Could you check a few things on this model? Use its own coordinates, in mm. A direction names the side the tool comes from. Round coordinates to 2 decimals unless told otherwise and drop trailing zeros. Loops run counter-clockwise (first coordinate to the right, second up) from the corner with the lowest first, then second, coordinate; pieces in that order, holes last. Notation, with made-up numbers: M 31.25,75.5 L 74.25,75.5 A21 cw 74.25,86.5 Z; hole C 35.25,55 d8. An arc over 180 degrees is marked long. One line per item, written item: value. Start each with the question number.
Q1. Imagine slicing it at A-A (z = -1.5). Please give me the cut outline in (x, y), then the cut area to 3 significant figures.
Q2. Imagine slicing it at C-C (z = 6.5). Please give me the cut outline in (x, y), then the cut area to 3 significant figures.
Q3. Which directions (+Z, -Z, +X, -X, +Y, -Y) give clear straight access to the entire face, cutting with the end or side of a thin tool? Please do faces 5 (the face through (-5.3, -0.1, 4.2)), 6 (the face through (-2, 3, -6)), 7 (the face through (15.25, 1, 0)), 8 (the face through (-12, 4, 7)), 9 (the face through (-0.52, 0.73, 0.03)).
Q4. Thinking about a two-plate mould opening in Z: for faces 1 (the face through (-5.62, -0.22, 6)), 2 (the face through (-5.3, -0.45, 7.01)), 3 (the face through (6, 5, 4)), 4 (the face through (0, 1, -8)), which applies, released by +Z, released by -Z, zero draft, split by the parting line, or undercut?
Q5. Please list where these lines run through material, in increasing order: line 1 along X through (y, z) = (2.5, -3.25); line 2 along Z through (x, y) = (-0.5, 1.5); line 3 along X through (y, z) = (5.5, 1.5).
Q6. I'm going to push flat-ended pins straight in: pin 1 Ø1.8 at (y, z) = (6.5, -1.5) entering from -X; pin 2 Ø1.2 at (x, z) = (14.5, 4) entering from +Y; pin 3 Ø2.5 at (x, y) = (-4, 0) entering from +Z; pin 4 Ø1.5 at (x, z) = (4.5, 0.5) entering from +Y. Where does each tip first touch, or does it pass through?
Q7. Imagine slicing it at B-B (x = -5.25). Please give me the cut outline in (y, z), then the cut area to 3 significant figures.
Q8. Imagine slicing it at D-D (x = 8). Please give me the cut outline in (y, z).
from build123d import *

# Parameters (mm, degrees)
BOSS_EXTRUDE1_DEPTH      = 2
BOSS_EXTRUDE1_DEPTH_BACK = 1
SKETCH1_W                = 30.5
SKETCH1_H                = 16
SKETCH2_W                = 2.4
SKETCH2_H                = 16
SKETCH2_W_2              = 26
SKETCH2_H_2              = 2
SKETCH2_W_3              = 2
SKETCH2_H_3              = 8.2
SKETCH2_W_4              = 2.279749354
BOSS_EXTRUDE2_DEPTH      = 2
SKETCH3_W                = 2
SKETCH3_H                = 8
BOSS_EXTRUDE3_DEPTH      = 6
SKETCH4_W                = 7
SKETCH4_H                = 4.5
CUT_EXTRUDE1_DEPTH       = 3
CUT_EXTRUDE2_DEPTH       = 7
CUT_EXTRUDE3_DEPTH       = 2
CHAMFER1_SIZE            = 2.5


with BuildPart() as part:
    # Sketch1 → Boss-Extrude1 (new, two sides: drawn at the far end of the back side and taken through both)
    with BuildSketch(Plane(origin=(0, 0, 0), x_dir=(1, 0, 0), z_dir=(0, 1, 0)).offset(-BOSS_EXTRUDE1_DEPTH_BACK)):
        Rectangle(SKETCH1_W, SKETCH1_H)
    extrude(amount=BOSS_EXTRUDE1_DEPTH + BOSS_EXTRUDE1_DEPTH_BACK)

    # Sketch2 → Boss-Extrude2 (add)
    with BuildSketch(Plane(origin=(0, 2, 0), x_dir=(1, 0, 0), z_dir=(0, 1, 0))):
        with Locations((14.05, 0)):
            Rectangle(SKETCH2_W, SKETCH2_H)
        with Locations((-2.25, 7)):
            Rectangle(SKETCH2_W_2, SKETCH2_H_2)
        with Locations((-2.25, -7)):
            Rectangle(SKETCH2_W_2, SKETCH2_H_2)
        with Locations((-14.25, 0.1)):
            Rectangle(SKETCH2_W_3, SKETCH2_H_3)
        with Locations((9.610125323, 0.1)):
            Rectangle(SKETCH2_W_4, SKETCH2_H_3)
    extrude(amount=BOSS_EXTRUDE2_DEPTH)

    # Sketch3 → Boss-Extrude3 (add)
    with BuildSketch(Plane(origin=(0, 2, 0), x_dir=(1, 0, 0), z_dir=(0, 1, 0))):
        with Locations((6.470250646, 0)):
            Rectangle(SKETCH3_W, SKETCH3_H)
    extrude(amount=BOSS_EXTRUDE3_DEPTH)

    # Sketch4 → Cut-Extrude1 (cut)
    with BuildSketch(Plane(origin=(0, 2, 0), x_dir=(1, 0, 0), z_dir=(0, 1, 0))):
        with Locations((-5.25, 0)):
            Rectangle(SKETCH4_W, SKETCH4_H)
    extrude(amount=-CUT_EXTRUDE1_DEPTH, mode=Mode.SUBTRACT)

    # Sketch5 → Cut-Extrude2 (cut)
    with BuildSketch(Plane(origin=(0, 0, 8), x_dir=(-1, 0, 0), z_dir=(0, 0, -1))):
        with BuildLine():
            Line((3.15, 2), (3.15, 4.2))
            Line((3.15, 4.2), (7.35, 4.2))
            Line((7.35, 4.2), (7.35, 2))
            ThreePointArc((7.35, 2), (5.25, -0.1), (3.15, 2))
        make_face()
    extrude(amount=CUT_EXTRUDE2_DEPTH, mode=Mode.SUBTRACT)

    # Sketch6 → Cut-Extrude3 (cut)
    with BuildSketch(Plane.XY.offset(8)):
        with BuildLine():
            Line((-7.7, 4), (-7.7, 2))
            ThreePointArc((-7.7, 2), (-5.25, -0.45), (-2.8, 2))
            Line((-2.8, 2), (-2.8, 4))
            Line((-2.8, 4), (-3, 4))
            Line((-3, 4), (-7.5, 4))
            Line((-7.5, 4), (-7.7, 4))
        make_face()
    extrude(amount=-CUT_EXTRUDE3_DEPTH, mode=Mode.SUBTRACT)

    # Chamfer1
    chamfer1_edges = [part.edges().sort_by_distance(p)[0] for p in [
        (-1.75, 2, 0),
        (-8.75, 2, 0),
    ]]
    chamfer(chamfer1_edges, length=CHAMFER1_SIZE)


solid = part.part
Report:
1. outline: M -15.25,-1 L -8.75,-1 L -8.75,-0.5 L -11.25,2 L -13.25,2 L -13.25,4 L -15.25,4 Z; M -1.75,-1 L 15.25,-1 L 15.25,4 L 12.85,4 L 12.85,2 L 10.75,2 L 10.75,4 L 8.47,4 L 8.47,2 L 7.47,2 L 7.47,8 L 5.47,8 L 5.47,2 L 0.75,2 L -1.75,-0.5 Z
1. area: 89.6 mm²
2. outline: M -15.25,-1 L 15.25,-1 L 15.25,4 L 12.85,4 L 12.85,2 L 10.75,2 L 10.75,4 L -2.8,4 L -2.8,2 A2.45 cw -7.7,2 L -7.7,4 L -15.25,4 Z
2. area: 129 mm²
3. face 5: +Z, +Y
3. face 6: -X, +Y
3. face 7: +Z, -Z, +X, +Y, -Y
3. face 8: +Z, -Z, +X, -X, +Y
3. face 9: +Y
4. face 1: released by +Z
4. face 2: zero draft
4. face 3: undercut
4. face 4: released by -Z
5. line 1: x = -15.25 to -13.25, 5.47 to 7.47, 8.47 to 10.75, 12.85 to 15.25
5. line 2: z = -8 to -2.25, 2.25 to 8
5. line 3: x = 5.47 to 7.47
6. pin 1: stops at x = 5.47
6. pin 2: stops at y = 4
6. pin 3: stops at z = 8
6. pin 4: stops at y = 2
7. outline: M -1,-8 L 4,-8 L 4,-6 L 2,-6 L 2,-2.25 L -1,-2.25 Z; M -1,2.25 L -0.1,2.25 L -0.1,6 L -0.45,6 L -0.45,8 L -1,8 Z
7. area: 25.7 mm²
8. outline: M -1,-8 L 4,-8 L 4,-6 L 2,-6 L 2,6 L 4,6 L 4,8 L -1,8 Z
